from build123d import *

# Parameters (mm, degrees)
F0_R     = 9.5
F1_DEPTH = 13
F2_R     = 5.08
F4_D     = 4


with BuildPart() as f1:
    # F0 (on Top) → F1 (new body)
    with BuildSketch(Plane.XY):
        Polygon((10.1788821743, 21.1366666282), (-10.1788821743, 21.1366666282), (-22.8717406344, 5.2203255477), (-18.3417118982, -14.6270271454), (0, -23.4599300611), (18.3417118982, -14.6270271454), (22.8717406344, 5.2203255477), align=None)
        Circle(F0_R, mode=Mode.SUBTRACT)
    extrude(amount=F1_DEPTH)

    # F2
    f2_edges = [f1.edges().sort_by_distance(p)[0] for p in [
        (-9.5, 0, 0),
        (-9.5, 0, 13),
        (-10.178882, 21.136667, 6.5),
        (-22.871741, 5.220326, 6.5),
        (-16.525311, 13.178496, 0),
        (-16.525311, 13.178496, 13),
        (-18.341712, -14.627027, 6.5),
        (-20.606726, -4.703351, 0),
        (-20.606726, -4.703351, 13),
        (0, -23.45993, 6.5),
        (-9.170856, -19.043479, 0),
        (-9.170856, -19.043479, 13),
        (18.341712, -14.627027, 6.5),
        (9.170856, -19.043479, 0),
        (9.170856, -19.043479, 13),
        (22.871741, 5.220326, 6.5),
        (20.606726, -4.703351, 0),
        (20.606726, -4.703351, 13),
        (10.178882, 21.136667, 6.5),
        (16.525311, 13.178496, 0),
        (16.525311, 13.178496, 13),
        (0, 21.136667, 0),
        (0, 21.136667, 13),
    ]]
    fillet(f2_edges, radius=F2_R)

    # F4 (through all)
    with Locations(Plane(origin=(0, 0, 0), x_dir=(1, 0, 0), z_dir=(0, 0, -1))):
        with Locations((0, -18.5665413737)):
            Hole(F4_D / 2)


solid = f1.part
Part model, mm, in its own coordinate system. Round coordinates to 2 decimals unless told otherwise and drop trailing zeros. Loops run counter-clockwise (first coordinate to the right, second up) from the corner with the lowest first, then second, coordinate; pieces in that order, holes last. Notation, with made-up numbers: (45, 64) - (82, 64) arc R16 ccw to (82, 73) - close; hole circle Ø6 at (-22, 61.5). An arc over 180 degrees is marked (long way). Answer as a JSON object with one key per item and string values.
Item 1: Wall check: L1, parallel to Y at x = 0, z = 4; L2, parallel to Y at x = 9, z = 2.75; L3, parallel to X at y = 2.5, z = 12.5. Give the ranges that are in metal, low to high.
Output:
{"L1": "-22.79 to -9.62, 9.62 to 16.57, 20.57 to 21.02", "L2": "-18.5 to -4.51, 4.51 to 20.39", "L3": "-19.29 to -12.13, 12.13 to 19.29"}
Item 2: Band-saw the part on C-C on x = -1. State how many separate pieces and enclosed holes the cut face has, plus the area to 3 significant figures.
Output:
{"separate pieces": "3", "enclosed holes": "0", "area": "241 mm2"}
Item 3: Band-saw the part on B-B on z = 6. List the corners of the cut face in (x, y), plus the area to 3 significant figures.
Output:
{"outline": "(-22.33, 2.84) - (-18.89, -12.24) arc R5.08 ccw to (-16.14, -15.69) - (-2.2, -22.4) arc R5.08 ccw to (2.2, -22.4) - (16.14, -15.69) arc R5.08 ccw to (18.89, -12.24) - (22.33, 2.84) arc R5.08 ccw to (21.35, 7.13) - (11.7, 19.22) arc R5.08 ccw to (7.73, 21.14) - (-7.73, 21.14) arc R5.08 ccw to (-11.7, 19.22) - (-21.35, 7.13) arc R5.08 ccw to start; hole circle Ø19 at (0, 0); hole circle Ø4 at (0, 18.57)", "area": "1,200 mm2"}
Item 4: Pin check, flat tips, straight feed: pin 1 (24.5 mm diameter, centred on x = 0, y = 0, fed in from -Z); pin 2 (3 mm diameter, centred on y = -14, z = 9.5, fed in from +X); pin 3 (2 mm diameter, centred on y = -9, z = 8.5, fed in from -X). Stop position of each tip, or through.
Output:
{"pin 1": "z = 0.57", "pin 2": "x = 18.69", "pin 3": "x = -19.84"}
Item 5: Pull direction X, two halves, no side cores. Call faces 1 (the face through (8.64, -17.691, 11.472)), 2 (the face through (0, -22.9, 6.5)), 3 (the face through (0.26, 16.584, 6.591)), 4 (the face through (-8.44, -17.79, 11.47)): pulls with the +X half, pulls with the -X half, needs draft (parallel to the pull), parting line crosses it, or undercut.
Output:
{"face 1": "pulls with the +X half", "face 2": "parting line crosses it", "face 3": "undercut", "face 4": "pulls with the -X half"}
Item 6: Band-saw the part on A-A on z = 2.5. List the corners of the cut face in (x, y), plus the area to 3 significant figures.
Output:
{"outline": "(-21.64, 2.99) - (-18.2, -12.09) arc R4.38 ccw to (-15.83, -15.05) - (-1.9, -21.76) arc R4.38 ccw to (1.9, -21.76) - (15.83, -15.05) arc R4.38 ccw to (18.2, -12.09) - (21.64, 2.99) arc R4.38 ccw to (20.8, 6.69) - (11.15, 18.79) arc R4.38 ccw to (7.73, 20.43) - (0.72, 20.43) arc R2 cw (long way) to (-0.72, 20.43) - (-7.73, 20.43) arc R4.38 ccw to (-11.15, 18.79) - (-20.8, 6.69) arc R4.38 ccw to start; hole circle Ø20.41 at (0, 0)", "area": "1,060 mm2"}
